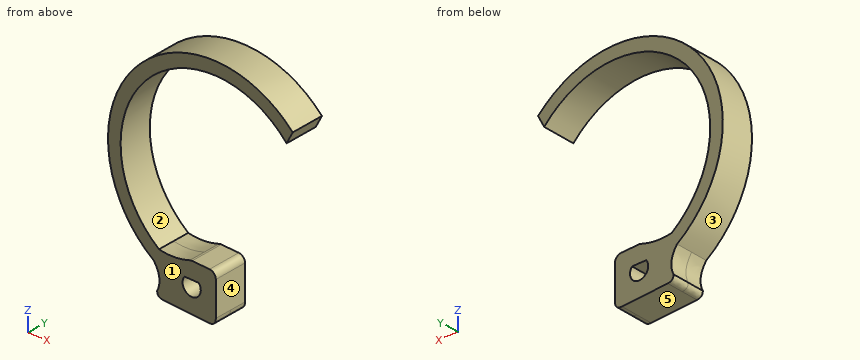
```python
from build123d import *

# Parameters (mm, degrees)
BOSS_EXTRUDE2_DEPTH     = 6.35
CUT_EXTRUDE1_DEPTH      = 0.254
CUT_EXTRUDE1_DEPTH_BACK = 13.208


with BuildPart() as part:
    # Sketch3 → Boss-Extrude2 (new, symmetric)
    with BuildSketch(Plane(origin=(0, 0, 0), x_dir=(1, 0, 0), z_dir=(0, 1, 0))):
        with BuildLine():
            Line((-52.600480424, -4.148495284), (-35.004351305, -3.195671149))
            add(Edge.make_bspline(
                [(-35.004351305, -3.195671149), (-32.391383355, -3.02906189), (-32.327012412, -5.731955445)],
                knots=[0, 0, 0, 1, 1, 1], degree=2))
            Line((-32.327012412, -5.731955445), (-32.327012412, -18.663867238))
            ThreePointArc((-32.327012412, -18.663867238), (-33.026692388, -20.3892504), (-34.730486544, -21.139973114))
            Line((-34.730486544, -21.139973114), (-41.447053807, -21.339967417))
            ThreePointArc((-41.447053807, -21.339967417), (-41.905677943, -21.312046914), (-42.351768326, -21.201960476))
            add(Edge.make_bspline(
                [(-42.351768326, -21.201960476), (-46.143088768, -19.892664891), (-50.094878971, -19.611768994), (-54.151069137, -20.370220418)],
                knots=[0.036271326, 0.036271326, 0.036271326, 0.036271326, 1, 1, 1, 1], degree=3))
            ThreePointArc((-54.151069137, -20.370220418), (-59.359137989, -74.344180893), (-5.134779033, -74.167301495))
            Line((-5.134779033, -74.167301495), (-2.773203125, -78.720626621))
            ThreePointArc((-2.773203125, -78.720626621), (-63.885313617, -76.526016755), (-56.177196586, -15.862260746))
            add(Edge.make_bspline(
                [(-54.866343349, -6.308912993), (-52.55640985, -10.963519078), (-56.177196586, -15.862260746)],
                knots=[0, 0, 0, 1, 1, 1], degree=2))
            add(Edge.make_bspline(
                [(-54.866343349, -6.308912993), (-54.833497461, -4.293658489), (-52.600480424, -4.148495284)],
                knots=[0, 0, 0, 1, 1, 1], degree=2))
        make_face()
    extrude(amount=BOSS_EXTRUDE2_DEPTH, both=True)

    # Sketch11 → Cut-Extrude1 (cut, two sides: drawn at the far end of the back side and taken through both)
    with BuildSketch(Plane(origin=(0, -6.35, 0), x_dir=(-1, 0, 0), z_dir=(0, -1, 0)).offset(-CUT_EXTRUDE1_DEPTH_BACK)):
        with BuildLine():
            Line((38.879229539, -15.029066428), (44.328612102, -15.029066428))
            ThreePointArc((44.328612102, -15.029066428), (41.603920821, -9.332237481), (38.879229539, -15.029066428))
        make_face()
    extrude(amount=CUT_EXTRUDE1_DEPTH + CUT_EXTRUDE1_DEPTH_BACK, mode=Mode.SUBTRACT)


solid = part.part
```
Geometry: final body of the model. Coordinates: model frame, mm. Face numbers are marked on the shaded views. A direction names the side the tool comes from. Round coordinates to 2 decimals unless told otherwise and drop trailing zeros. Order: outer loops, then holes, each group sorted by start corner. A loop starts at its lowest first (then second) coordinate and runs counter-clockwise, first axis right, second up. Notation, with made-up numbers: (65.5, 43) - (106.5, 43) arc R28 ccw to (106.5, 77) - close; hole circle Ø8 at (60.25, 74). An arc over 180 degrees is marked (long way). Write item = value, one per line. Start each with the question number.
Q1. Cut plane C-C on x = -21. Return the cut outline in (y, z), and give its area (3 significant figures).
Q2. Cut plane D-D on z = 31. Return the cut outline in (x, y).
Q3. Pin query (flat end, axial travel): pin 1 (4 mm diameter, centred on y = -3, z = 14.5, fed in from +X); pin 2 (2 mm diameter, centred on x = -47.5, y = -1.5, fed in from -Z); pin 3 (1.6 mm diameter, centred on x = -43, y = -1.5, fed in from -Z). Return the tip coordinate at first contact, or that it passes through.
Q4. Ray query, line 1 (Z direction, x = -43, y = -0.5); line 2 (X direction, y = 0.5, z = 49); line 3 (Z direction, x = -60.5, y = -2.25). Return the intervals inside material, ascending. Write a range as from..to.
Q5. Cut plane B-B on x = -62.5. Return the cut outline in (y, z), and give its area (3 significant figures).
Q6. Cut plane A-A on z = 80.5. Return the cut outline in (x, y).
Q7. Pull-direction query (Z, two-part tool) for the marked faces 1, 2 and 3; classes: +Z half, -Z half, draft (parallel to the pull), parting line (faces both ways), or undercut.
Q8. Access query for the marked faces 4 and 5. Directions: +Z, -Z, +X, -X, +Y, -Y. A direction counts if a zero-diameter tool reaches every point of the face in a straight line with its end or side. Return the directions, or none.
Outcome:
q1.outline = (-6.35, 84.49) - (6.35, 84.49) - (6.35, 89.55) - (-6.35, 89.55) - close
q1.area = 64.3 mm^2
q2.outline = (-69.27, -6.35) - (-63.75, -6.35) - (-63.75, 6.35) - (-69.27, 6.35) - close
q3.pin_1 = -32.33
q3.pin_2 = 3.82
q3.pin_3 = 3.59
q4.line_1 = 3.63..9.62, 15.03..20.99, 84.69..89.73
q4.line_2 = -73.73..-68.89
q4.line_3 = 19.37..26.4, 73.03..80.06
q5.outline = (-6.35, 21.35) - (6.35, 21.35) - (6.35, 29.05) - (-6.35, 29.05) - close; (-6.35, 70.38) - (6.35, 70.38) - (6.35, 78.08) - (-6.35, 78.08) - close
q5.area = 196 mm^2
q6.outline = (-60.02, -6.35) - (-52.07, -6.35) - (-52.07, 6.35) - (-60.02, 6.35) - close; (-12.59, -6.35) - (-4.63, -6.35) - (-4.63, 6.35) - (-12.59, 6.35) - close
q7.face_1 = draft
q7.face_2 = undercut
q7.face_3 = parting line
q8.face_4 = -Z, +X, +Y, -Y
q8.face_5 = -Z, -X, +Y, -Y
